Work out the finished part from the listing and answer in its coordinate system (mm). Round coordinates to 2 decimals unless told otherwise and drop trailing zeros. Write each loop counter-clockwise with the first axis right and the second up, starting at its lowest first coordinate (ties: lowest second). Pieces come first, ordered by that corner, then holes. Notation, with made-up numbers: (-29, 3) -> (-16, 3) arc R10 cw to (-16, 14) -> close; hole circle Ø9 at (4.5, 7). An arc over 180 degrees is marked (long way). Answer as a JSON object with one key per item and string values. Group by question number.
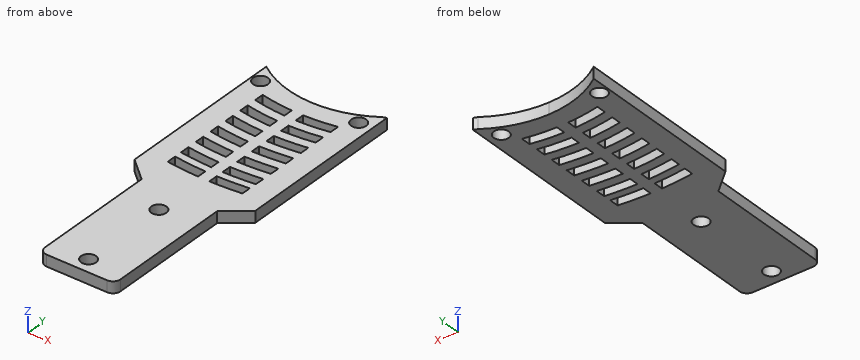
from build123d import *

# Parameters (mm, degrees)
SKETCH1_W                    = 20
SKETCH1_H                    = 35
BOSS_EXTRUDE1_DEPTH          = 3
FILLET5_R                    = 2
F_97_0_0059_DIAMETER_HOLE2_D = 3.000000096
F_97_0_0059_DIAMETER_HOLE4_D = 3.000000096
F_97_0_0059_DIAMETER_HOLE6_D = 3.000000096
F_97_0_0059_DIAMETER_HOLE7_D = 3.000000096
CUT_EXTRUDE1_DEPTH           = 3
BOSS_EXTRUDE3_START          = -3
SKETCH17_R                   = 1.500000048
BOSS_EXTRUDE3_DEPTH          = 3
CUT_EXTRUDE3_START           = -3
CUT_EXTRUDE3_DEPTH           = 3
SKETCH19_R                   = 2
CUT_EXTRUDE4_DEPTH           = 10
SKETCH20_R                   = 2
CUT_EXTRUDE6_DEPTH           = 10


with BuildPart() as part:
    # Sketch1 → Boss-Extrude1 (new body)
    with BuildSketch(Plane.XY):
        with BuildLine():
            Line((-16, 22.5), (-16, -22.5))
            Line((-16, -22.5), (16, -22.5))
            Line((16, -22.5), (16, 22.5))
            ThreePointArc((16, 22.5), (0, 19.418681543), (-16, 22.5))
        make_face()
        with Locations((-0.22513797, -45.024704694)):
            Rectangle(SKETCH1_W, SKETCH1_H)
        Polygon((9.77486203, -27.524704694), (-10.22513797, -27.524704694), (-16, -22.5), (16, -22.5), align=None)
    extrude(amount=BOSS_EXTRUDE1_DEPTH)

    # Fillet5
    fillet5_edges = [part.edges().sort_by_distance(p)[0] for p in [
        (9.77486203, -62.524704694, 1.5),
        (-10.22513797, -62.524704694, 1.5),
    ]]
    fillet(fillet5_edges, radius=FILLET5_R)

    # #97 (0.0059) Diameter Hole2 (through all)
    with Locations(Plane(origin=(-0.22513797, -57.524704694, 3), x_dir=(1, 0, 0), z_dir=(0, 0, 1))):
        with Locations((0, 0)):
            Hole(F_97_0_0059_DIAMETER_HOLE2_D / 2)

    # #97 (0.0059) Diameter Hole4 (through all)
    with Locations(Plane(origin=(-0.22513797, -32.524704694, 3), x_dir=(1, 0, 0), z_dir=(0, 0, 1))):
        with Locations((0, 0)):
            Hole(F_97_0_0059_DIAMETER_HOLE4_D / 2)

    # #97 (0.0059) Diameter Hole6 (through all)
    with Locations(Plane(origin=(-13.971666748, 19.647656364, 3), x_dir=(1, 0, 0), z_dir=(0, 0, 1))):
        with Locations((0, 0)):
            Hole(F_97_0_0059_DIAMETER_HOLE6_D / 2)

    # #97 (0.0059) Diameter Hole7 (through all)
    with Locations(Plane(origin=(13.932427901, 19.6445071, 3), x_dir=(1, 0, 0), z_dir=(0, 0, 1))):
        with Locations((0, 0)):
            Hole(F_97_0_0059_DIAMETER_HOLE7_D / 2)

    # Sketch15 → Cut-Extrude1 (cut)
    with BuildSketch(Plane.XY.offset(3)):
        with BuildLine():
            ThreePointArc((10, 13.510205144), (5.771168674, 12.834180646), (1.5, 12.522505065))
            Line((1.5, 12.522505065), (1.5, 10.021432946))
            ThreePointArc((1.5, 10.021432946), (5.769166403, 10.317946389), (10, 10.96117968))
            Line((10, 10.96117968), (10, 13.510205144))
        make_face()
        with BuildLine():
            Line((-1.5, 10.021432946), (-1.5, 12.522505065))
            ThreePointArc((-1.5, 12.522505065), (-5.771168674, 12.834180646), (-10, 13.510205144))
            Line((-10, 13.510205144), (-10, 10.96117968))
            ThreePointArc((-10, 10.96117968), (-5.769166403, 10.317946389), (-1.5, 10.021432946))
        make_face()
        with BuildLine():
            Line((-1.5, 5.019568547), (-1.5, 7.52045835))
            ThreePointArc((-1.5, 7.52045835), (-5.767436702, 7.803229767), (-10, 8.416730868))
            Line((-10, 8.416730868), (-10, 5.876241735))
            ThreePointArc((-10, 5.876241735), (-5.765932035, 5.289825837), (-1.5, 5.019568547))
        make_face()
        with BuildLine():
            ThreePointArc((10, 8.416730868), (5.767436702, 7.803229767), (1.5, 7.52045835))
            Line((1.5, 7.52045835), (1.5, 5.019568547))
            ThreePointArc((1.5, 5.019568547), (5.765932035, 5.289825837), (10, 5.876241735))
            Line((10, 5.876241735), (10, 8.416730868))
        make_face()
        with BuildLine():
            Line((-1.5, 0.018002593), (-1.5, 2.518752931))
            ThreePointArc((-1.5, 2.518752931), (-5.764614839, 2.777565222), (-10, 3.339202169))
            Line((-10, 3.339202169), (-10, 0.805186604))
            ThreePointArc((-10, 0.805186604), (-5.763455098, 0.266306671), (-1.5, 0.018002593))
        make_face()
        with BuildLine():
            ThreePointArc((10, 3.339202169), (5.764614839, 2.777565222), (1.5, 2.518752931))
            Line((1.5, 2.518752931), (1.5, 0.018002593))
            ThreePointArc((1.5, 0.018002593), (5.763455098, 0.266306671), (10, 0.805186604))
            Line((10, 0.805186604), (10, 3.339202169))
        make_face()
        with BuildLine():
            Line((-1.5, -4.983331275), (-1.5, -2.482690003))
            ThreePointArc((-1.5, -2.482690003), (-5.762428595, -2.244068583), (-10, -1.726162893))
            Line((-10, -1.726162893), (-10, -4.255149614))
            ThreePointArc((-10, -4.255149614), (-5.761515611, -4.753661148), (-1.5, -4.983331275))
        make_face()
        with BuildLine():
            ThreePointArc((9.981645143, -1.729018054), (5.753177309, -2.244891311), (1.5, -2.482690003))
            Line((1.5, -2.482690003), (1.5, -4.983331275))
            ThreePointArc((1.5, -4.983331275), (5.738725767, -4.755609629), (9.95475653, -4.261911465))
            Line((9.95475653, -4.261911465), (9.981645143, -1.729018054))
        make_face()
        with BuildLine():
            Line((-1.5, -9.984481098), (-1.5, -7.483926726))
            ThreePointArc((-1.5, -7.483926726), (-5.760699953, -7.262556834), (-10, -6.782032303))
            Line((-10, -6.782032303), (-10, -9.307033082))
            ThreePointArc((-10, -9.307033082), (-5.759968225, -9.770829288), (-1.5, -9.984481098))
        make_face()
        with BuildLine():
            ThreePointArc((9.927893429, -6.792401691), (5.724398551, -7.265544943), (1.5, -7.483926726))
            Line((1.5, -7.483926726), (1.5, -9.984481098))
            ThreePointArc((1.5, -9.984481098), (5.710178647, -9.774780247), (9.901053138, -9.320743151))
            Line((9.901053138, -9.320743151), (9.927893429, -6.792401691))
        make_face()
        with BuildLine():
            Line((-1.5, -14.985482511), (-1.5, -12.4849985))
            ThreePointArc((-1.5, -12.4849985), (-5.759309265, -12.278542088), (-10, -11.830343737))
            Line((-10, -11.830343737), (-10, -14.352130745))
            ThreePointArc((-10, -14.352130745), (-5.758713712, -14.78575041), (-1.5, -14.985482511))
        make_face()
        with BuildLine():
            Line((-1.5, -19.48627934), (-1.5, -16.985847797))
            ThreePointArc((-1.5, -16.985847797), (-5.758277571, -16.791186392), (-10, -16.368561544))
            Line((-10, -16.368561544), (-10, -18.887959798))
            ThreePointArc((-10, -18.887959798), (-5.757777051, -19.297603898), (-1.5, -19.48627934))
        make_face()
        with BuildLine():
            ThreePointArc((9.82600299, -16.390428223), (5.67082155, -16.797489134), (1.5, -16.985847797))
            Line((1.5, -16.985847797), (1.5, -19.48627934))
            ThreePointArc((1.5, -19.48627934), (5.656897905, -19.304642326), (9.799230566, -18.912376702))
            Line((9.799230566, -18.912376702), (9.82600299, -16.390428223))
        make_face()
        with BuildLine():
            ThreePointArc((9.874233328, -11.847155401), (5.69605187, -12.283387146), (1.5, -12.4849985))
            Line((1.5, -12.4849985), (1.5, -14.985482511))
            ThreePointArc((1.5, -14.985482511), (5.682006317, -14.791427754), (9.847431975, -14.371828933))
            Line((9.847431975, -14.371828933), (9.874233328, -11.847155401))
        make_face()
    extrude(amount=-CUT_EXTRUDE1_DEPTH, mode=Mode.SUBTRACT)

    # Sketch17 → Boss-Extrude3 (add)
    with BuildSketch(Plane.XY.offset(3).offset(BOSS_EXTRUDE3_START)):
        with Locations((-0.22513797, -57.524704694)):
            Circle(SKETCH17_R)
        with Locations((-0.22513797, -32.524704694)):
            Circle(SKETCH17_R)
        with Locations((-13.971666748, 19.647656364)):
            Circle(SKETCH17_R)
        with Locations((13.932427901, 19.6445071)):
            Circle(SKETCH17_R)
    extrude(amount=BOSS_EXTRUDE3_DEPTH)

    # Sketch18 → Cut-Extrude3 (cut)
    with BuildSketch(Plane.XY.offset(3).offset(CUT_EXTRUDE3_START)):
        with BuildLine():
            ThreePointArc((-16, 22.5), (-8.51081333, 18.724422317), (-0.22513797, 17.424234775))
            Line((-0.22513797, 17.424234775), (-0.22513797, 19.419269819))
            ThreePointArc((-0.22513797, 19.419269819), (-8.257511741, 20.217456322), (-16, 22.5))
        make_face()
        with BuildLine():
            Line((-0.22513797, 19.419269819), (-0.22513797, 17.424234775))
            ThreePointArc((-0.22513797, 17.424234775), (7.738274372, 18.622946482), (14.995922473, 22.11284475))
            ThreePointArc((14.995922473, 22.11284475), (7.507186902, 20.077810702), (-0.22513797, 19.419269819))
        make_face()
    extrude(amount=CUT_EXTRUDE3_DEPTH, mode=Mode.SUBTRACT)

    # Sketch19 → Cut-Extrude4 (cut)
    with BuildSketch(Plane.XY.offset(3)):
        with Locations((-0.22513797, -34.524704694)):
            Circle(SKETCH19_R)
        with Locations((-0.22513797, -58.524704694)):
            Circle(SKETCH19_R)
    extrude(amount=-CUT_EXTRUDE4_DEPTH, mode=Mode.SUBTRACT)

    # Sketch20 → Cut-Extrude6 (cut)
    with BuildSketch(Plane(origin=(0, 0, 0), x_dir=(-1, 0, 0), z_dir=(0, 0, -1))):
        with Locations((13.562993481, 17.426344688)):
            Circle(SKETCH20_R)
        with Locations((-12.437006519, 17.426344688)):
            Circle(SKETCH20_R)
    extrude(amount=-CUT_EXTRUDE6_DEPTH, mode=Mode.SUBTRACT)


solid = part.part
1) A cutting plane is placed at A-A on x = -5.5. State how many separate pieces and enclosed holes the cut face has, plus the area to 3 significant figures.
2) A cutting plane is placed at B-B on y = -45. Determine the outline of the cut face in (x, z), plus the area to 3 significant figures.
3) Straight lines are drawn through the part: L1, parallel to X at y = -13.5, z = 2.45; L2, parallel to X at y = -18.5, z = 2.6; L3, parallel to X at y = -40, z = 2.45. For each, find the intervals that lie inside material, in ascending order.
Established:
{
 "1": {"separate pieces": "8", "enclosed holes": "0", "area": "189 mm²"},
 "2": {"outline": "(-10.23, 0) -> (9.77, 0) -> (9.77, 3) -> (-10.23, 3) -> close", "area": "60.0 mm²"},
 "3": {"L1": "x = -16 to -10, -1.5 to 1.5, 9.86 to 16", "L2": "x = -16 to -10, -1.5 to 1.5, 9.8 to 16", "L3": "x = -10.23 to 9.77"}
}
